Job drawing, mm, ordinate dimensions from the low corner. One solid piece. A direction names the side the tool comes from. Round coordinates to 2 decimals unless told otherwise and drop trailing zeros. Loops run counter-clockwise (first coordinate to the right, second up) from the corner with the lowest first, then second, coordinate; pieces in that order, holes last.
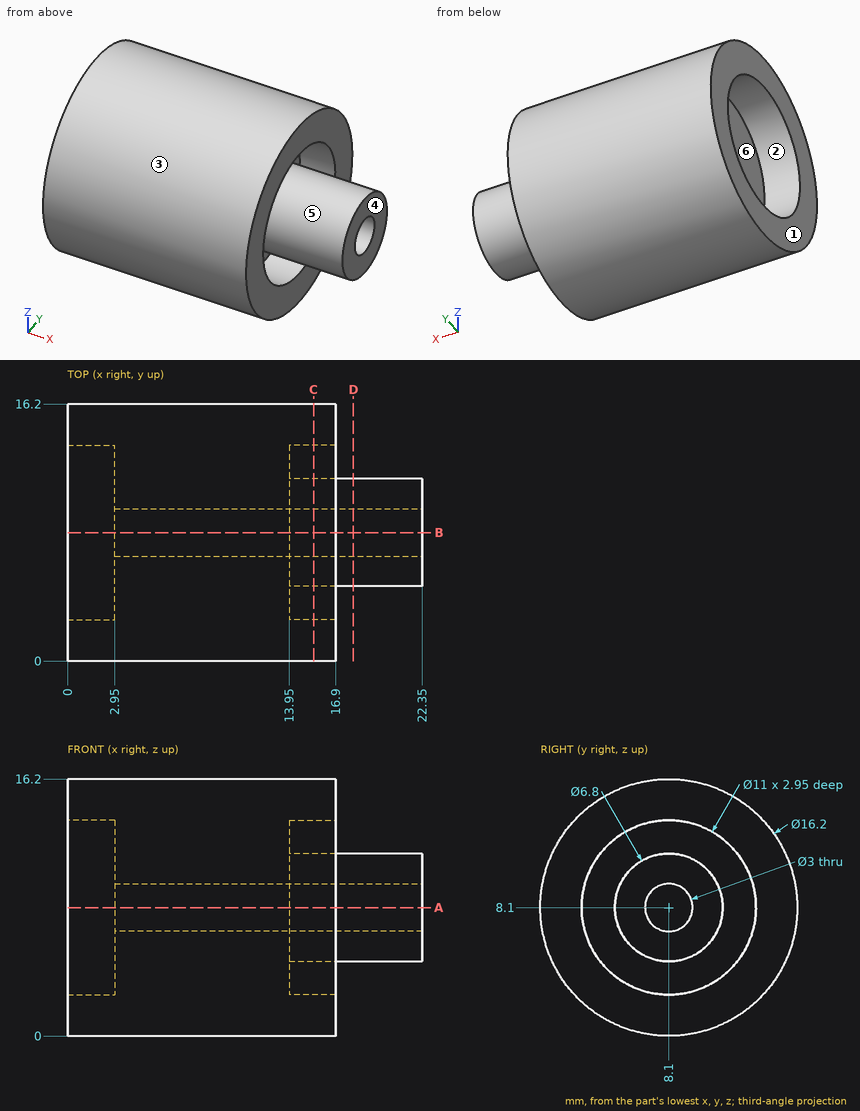
Item 1: Cut at C-C, the plane x = 15.5. Give the cut face in (y, z), plus the area to 3 significant figures.
Answers follow:
outline: circle Ø16.2 at (8.1, 8.1); circle Ø6.8 at (8.1, 8.1); hole circle Ø11 at (8.1, 8.1); hole circle Ø3 at (8.1, 8.1)
area: 140 mm2
Item 2: Cut at D-D, the plane x = 18. Give the cut face in (y, z).
Answers follow:
outline: circle Ø6.8 at (8.1, 8.1); hole circle Ø3 at (8.1, 8.1)
Item 3: Probe line 1 (Y direction, x = 15.65, z = 8.1); line 2 (Y direction, x = 0.9, z = 8.1); line 3 (Y direction, x = 10.75, z = 8.1). List the from-to ranges inside material, lowest first.
Answers follow:
line 1: y = 0 to 2.6, 4.7 to 6.6, 9.6 to 11.5, 13.6 to 16.2
line 2: y = 0 to 2.6, 13.6 to 16.2
line 3: y = 0 to 6.6, 9.6 to 16.2
Item 4: Cut at A-A, the plane z = 8.1. Give the cut face in (x, y).
Answers follow:
outline: (0, 0) - (16.9, 0) - (16.9, 2.6) - (13.95, 2.6) - (13.95, 4.7) - (22.35, 4.7) - (22.35, 6.6) - (2.95, 6.6) - (2.95, 2.6) - (0, 2.6) - close; (0, 13.6) - (2.95, 13.6) - (2.95, 9.6) - (22.35, 9.6) - (22.35, 11.5) - (13.95, 11.5) - (13.95, 13.6) - (16.9, 13.6) - (16.9, 16.2) - (0, 16.2) - close
Item 5: Flat gauge pins, fed straight in: P1, Ø1.5, axis at x = 4, y = 13.5, coming from the +Z side; P2, Ø1, axis at x = 10, y = 9, coming from the +Z side; P3, Ø1.5, axis at y = 6, z = 6.5, coming from the -X side. Where does each tip first touch, or does it go through?
Answers follow:
P1: stops at z = 14.73
P2: stops at z = 16.19
P3: stops at x = 2.95
Item 6: 3-axis set-ups, long thin cutter, end or side, ignore diameter. For the marked faces 4, 5 and 6: which of +Z, -Z, +X, -X, +Y, -Y reach the whole face in a straight line?
Answers follow:
face 4: +Z, -Z, +X, +Y, -Y
face 5: +X
face 6: -X
Item 7: Two-plate mould, pull along Z, no slides. Class the marked faces 1, 2 and 3: released by +Z, released by -Z, zero draft, split by the parting line, or undercut.
Answers follow:
face 1: zero draft
face 2: undercut
face 3: split by the parting line
